Build history of the part. All positions in model axes, mm. A direction names the side the tool comes from. Round coordinates to 2 decimals unless told otherwise and drop trailing zeros. Write each loop counter-clockwise with the first axis right and the second up, starting at its lowest first coordinate (ties: lowest second). Pieces come first, ordered by that corner, then holes. Notation, with made-up numbers: M 23.25,89.5 L 81.25,89.5 A26 cw 81.25,127.5 Z; hole C -25,20.5 d6. An arc over 180 degrees is marked long. Write item = value, one per line. Start each with the question number.
Q1. Band-saw the part on B-B on x = -196.5. Write the cut outline in (y, z).
Q2. Band-saw the part on C-C on y = 207. Write the cut outline in (x, z), plus the area to 3 significant figures.
Q3. Probe L1, parallel to X at y = 94, z = -3; L2, parallel to Z at x = 1, y = -71; L3, parallel to Z at x = 267, y = 197. List the from-to ranges inside material, lowest first.
Q4. Pull direction X, two halves, no side cores. Call faces 3 (the flat face through (-5, 3, -254)), 4 (the flat face through (-355.6, 3, 4)), 5 (the flat face through (-5, 5, -251.46)): released by +X, released by -X, zero draft, split by the parting line, or undercut.
Q5. Band-saw the part on A-A on y = -110. Write the cut outline in (x, z), plus the area to 3 significant figures.
Q6. Drop flat-ended pins along their axis: P1, Ø3, axis at x = 112, z = -78, coming from the +Y side; P2, Ø3, axis at x = -1, z = 253, coming from the +Y side. Give the stop position or say it passes through.
Q7. Tool access for faces 1 (the flat face through (355.6, 3, 4)), 2 (the flat face through (-5, -238.76, -4)): list every direction of +Z, -Z, +X, -X, +Y, -Y with a clear straight run to the whole face (end or side of a thin tool).
```python
from build123d import *

# Parameters (mm, degrees)
SKETCH1_W           = 711.2
SKETCH1_H           = 508
BOSS_EXTRUDE1_DEPTH = 241.3
SHELL1_T            = -2.54
CUT_EXTRUDE1_REACH  = 510
SKETCH2_W           = 706.12
SKETCH2_H           = 127


with BuildPart() as part:
    # Sketch1 → Boss-Extrude1 (new body, symmetric)
    with BuildSketch(Plane(origin=(0, 0, 0), x_dir=(1, 0, 0), z_dir=(0, 1, 0))):
        Rectangle(SKETCH1_W, SKETCH1_H)
    extrude(amount=BOSS_EXTRUDE1_DEPTH, both=True)

    # Shell1
    shell1_openings = [part.faces().sort_by_distance(p)[0] for p in [
        (0, 241.3, 0),
    ]]
    offset(amount=SHELL1_T, openings=shell1_openings, kind=Kind.INTERSECTION)

    # Sketch2 → Cut-Extrude1 (cut, up to next)
    with BuildSketch(Plane.XY.offset(254), mode=Mode.PRIVATE) as cut_extrude1_sk1:
        with Locations((0, 177.8)):
            Rectangle(SKETCH2_W, SKETCH2_H)
    cut_extrude1_tool1 = extrude(cut_extrude1_sk1.sketch, amount=-CUT_EXTRUDE1_REACH, mode=Mode.PRIVATE) & part.part
    add(cut_extrude1_tool1.solids().sort_by_distance((0, 177.8, 254))[0], mode=Mode.SUBTRACT)


solid = part.part
```
Conclusion:
q1.outline = M -241.3,-254 L 241.3,-254 L 241.3,-251.46 L -238.76,-251.46 L -238.76,251.46 L 114.3,251.46 L 114.3,254 L -241.3,254 Z
q2.outline = M -355.6,-254 L 355.6,-254 L 355.6,254 L 353.06,254 L 353.06,-251.46 L -353.06,-251.46 L -353.06,254 L -355.6,254 Z
q2.area = 4,370 mm^2
q3.L1 = -355.6 to -353.06, 353.06 to 355.6
q3.L2 = -254 to -251.46, 251.46 to 254
q3.L3 = -254 to -251.46
q4.face_3 = zero draft
q4.face_4 = released by -X
q4.face_5 = undercut
q5.outline = M -355.6,-254 L 355.6,-254 L 355.6,254 L -355.6,254 Z; hole M -353.06,-251.46 L 353.06,-251.46 L 353.06,251.46 L -353.06,251.46 Z
q5.area = 6,170 mm^2
q6.P1 = -238.76
q6.P2 = 114.3
q7.face_1 = +Z, -Z, +X, +Y, -Y
q7.face_2 = +Y
